Autodesk Inventor part; units mm, degrees
ref_plane "YZ Plane" through (0, 0, 0) normal (1, 0, 0) x (0, 1, 0)
ref_plane "XZ Plane" through (0, 0, 0) normal (0, 1, 0) x (-1, 0, 0)
ref_plane "XY Plane" through (0, 0, 0) normal (0, 0, 1) x (1, 0, 0)
sketch "Sketch1" plane through (0, 0, 0) normal (0, 0, 1) x (1, 0, 0)
  circle A0 centre (0, 0) radius 6
  line L0 (0, -2) -> (0, 80) construction
  line L1 (4, -2) -> (4, 80)
  line L2 (-4, 80) -> (-4, -2)
  arc A1 (-4, -2) -> (4, -2) centre (0, -2) ccw
  arc A2 (4, 80) -> (-4, 80) centre (0, 80) ccw
  point P0 (0, 39)
  dimension "d0" = 12
  dimension "d1" = 8
  dimension "d2" = 80
extrude "Extrusion1" add sketch "Sketch1" along normal mid plane 2.8
sketch "Sketch2" plane through (0, 0, 1.4) normal (0, 0, 1) x (1, 0, 0)
  arc A0 (4, 80) -> (-4, 80) centre (0, 80) ccw construction
  arc A1 (-4, 4.4721) -> (4, 4.4721) centre (0, 0) ccw construction
  circle A2 centre (0, 0) radius 1.75
  circle A3 centre (0, 80) radius 1.75
  line L0 (0, 12.7) -> (0, 5.7) construction
  line L1 (-1.3, 11.4) -> (-1.3, 7)
  line L2 (1.3, 7) -> (1.3, 11.4)
  arc A4 (1.3, 11.4) -> (-1.3, 11.4) centre (0, 11.4) ccw
  arc A5 (-1.3, 7) -> (1.3, 7) centre (0, 7) ccw
  point P0 (0, 9.2)
  dimension "d5" = 7
  dimension "d6" = 2.6
  dimension "d7" = 7
  dimension "d8" = 3.5
  dimension "d9" = 3.5
extrude "Extrusion2" cut sketch "Sketch2" against normal through all contours A2 | A3
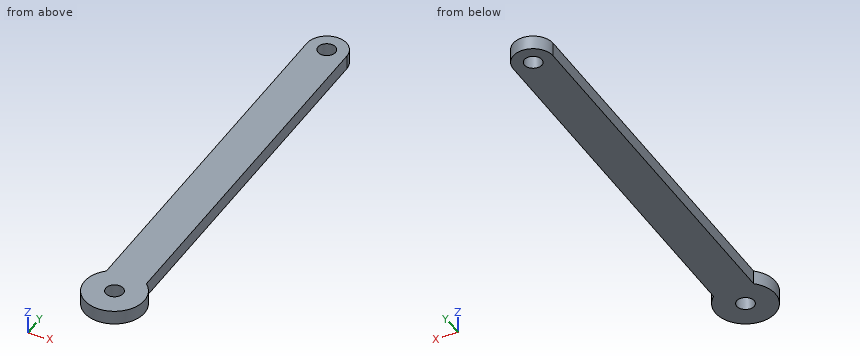
Verification items for the finished model (mm, model axes). Coordinates: 2 decimals unless noted, no trailing zeros. Write each loop counter-clockwise with the first axis right and the second up, starting at its lowest first coordinate (ties: lowest second). Pieces come first, ordered by that corner, then holes. Notation, with made-up numbers: (-5.75, 58) - (12.25, 58) arc R22 cw to (12.25, 67) - close; hole circle Ø9 at (78, -4.75). An arc over 180 degrees is marked (long way). One line per question, with ' | ' between items. Start each with the question number.
1. Section check C-C (z = -0.2). Enter the section's corners in (x, y).
2. Section check D-D (y = 55.5). Enter the section's corners in (x, z), plus the area to 3 significant figures.
3. Material ranges on line 1 along Y through (x, z) = (0, 0.85); line 2 along X through (y, z) = (80, -0.15); line 3 along X through (y, z) = (12, 0.05), recorded low to high.
4. Gauge pin test, flat ends, axial feed: P1, Ø1, axis at y = 50.5, z = 0, coming from the -X side; P2, Ø1.5, axis at x = -2.5, z = 0, coming from the +Y side; P3, Ø1, axis at x = -3.5, z = 1, coming from the +Y side. Record the tip position at first contact, or that the pin passes through.
5. Section check B-B (y = 0). Enter the section's corners in (x, z).
6. Section check A-A (x = 0). Enter the section's corners in (y, z).
Computed values:
1) outline: (-4, 4.47) arc R6 ccw (long way) to (4, 4.47) - (4, 80) arc R4 ccw to (-4, 80) - close; hole circle Ø3.5 at (0, 0); hole circle Ø3.5 at (0, 80)
2) outline: (-4, -1.4) - (4, -1.4) - (4, 1.4) - (-4, 1.4) - close | area: 22.4 mm²
3) line 1: -6 to -1.75, 1.75 to 78.25, 81.75 to 84 | line 2: -4 to -1.75, 1.75 to 4 | line 3: -4 to 4
4) P1: x = -4 | P2: y = 83.6 | P3: y = 82.65
5) outline: (-6, -1.4) - (-1.75, -1.4) - (-1.75, 1.4) - (-6, 1.4) - close; (1.75, -1.4) - (6, -1.4) - (6, 1.4) - (1.75, 1.4) - close
6) outline: (-6, -1.4) - (-1.75, -1.4) - (-1.75, 1.4) - (-6, 1.4) - close; (1.75, -1.4) - (78.25, -1.4) - (78.25, 1.4) - (1.75, 1.4) - close; (81.75, -1.4) - (84, -1.4) - (84, 1.4) - (81.75, 1.4) - close
